Build history of the part. All positions in model axes, mm. A direction names the side the tool comes from. Give positions to 0.01 mm unless a question says otherwise; leave off trailing zeros. Loops run counter-clockwise (first coordinate to the right, second up) from the corner with the lowest first, then second, coordinate; pieces in that order, holes last. Notation, with made-up numbers: M 12.25,-24 L 52.25,-24 A29 cw 52.25,0 Z; hole C -38,-32.75 d10. An arc over 180 degrees is marked long. Answer as a JSON object with one key per item and string values. Group by question number.
1. Slice it at B-B (z = -64). List the corners of the cut face in (x, y).
2. Drop flat-ended pins along their axis: pin 1 Ø5 at (x, y) = (-1, 17.5) entering from -Z; pin 2 Ø8 at (y, z) = (1, -7.5) entering from -X; pin 3 Ø10.5 at (y, z) = (-20.5, -50.5) entering from +X; pin 4 Ø1 at (y, z) = (-5.5, -8.5) entering from +X. Give the stop position or say it passes through.
3. 3-axis set-ups, long thin cutter, end or side, ignore diameter. For faces 4 (the face through (6, -19, -54)), 5 (the face through (-3.525, -20.938, -54.072)), 6 (the face through (14, 0, 10)), 7 (the face through (-7.542, -23.397, -77.292)): which of +Z, -Z, +X, -X, +Y, -Y reach the whole face in a straight line?
4. Slice it at A-A (x = 20). List the corners of the cut face in (y, z), then the cut area to 3 significant figures.
5. Drill centre lines: line 1 along Z through (x, y) = (-4, -9.5); line 2 along X through (y, z) = (6.5, -2.5); line 3 along Z through (x, y) = (-21, -20.5). Where is each one in solid material? Low to high. Write a range as [from, to].
6. Mould opens along Z. For faces 1 (the face through (12.432, -8.508, -14.781)), 2 (the face through (-0.21, -10.896, -15.698)), 3 (the face through (25, 0, 0)) say: released by +Z, released by -Z, zero draft, split by the parting line, or undercut.
from build123d import *

# Parameters (mm, degrees)
BOSS_EXTRUDE1_DEPTH      = 25
BOSS_EXTRUDE1_DEPTH_BACK = 10
SKETCH1_R                = 10
SKETCH2_R                = 12.5
BOSS_EXTRUDE2_DEPTH      = 25
BOSS_EXTRUDE3_DEPTH      = 15
BOSS_EXTRUDE3_DEPTH_BACK = 15
CUT_EXTRUDE1_DEPTH       = 15
BOSS_EXTRUDE4_DEPTH      = 3.175
CUT_EXTRUDE2_DEPTH       = 96.96083651
CUT_EXTRUDE2_DEPTH_BACK  = 96.96083651
SKETCH10_R               = 5
CUT_EXTRUDE3_DEPTH       = 10


with BuildPart() as part:
    # Sketch1 → Boss-Extrude1 (new, two sides: drawn at the far end of the back side and taken through both)
    with BuildSketch(Plane(origin=(0, 0, 0), x_dir=(0, 0, -1), z_dir=(1, 0, 0)).offset(-BOSS_EXTRUDE1_DEPTH_BACK)):
        Circle(SKETCH1_R)
    extrude(amount=BOSS_EXTRUDE1_DEPTH + BOSS_EXTRUDE1_DEPTH_BACK)

    # Sketch2 → Boss-Extrude2 (add, symmetric)
    with BuildSketch(Plane(origin=(-10, 0, 0), x_dir=(0.9848069802426886, -0.173652560203633, 1.5808464272800858e-08), z_dir=(0.17364817766692736, 0.9847821256419462, -0.007104604780387524))):
        with Locations(Location((0, 0, 0), (0, 0, 180.000000906))):
            Circle(SKETCH2_R)
    extrude(amount=BOSS_EXTRUDE2_DEPTH, both=True)

    # Sketch5 → Boss-Extrude3 (add, two sides: drawn at the far end of the back side and taken through both)
    with BuildSketch(Plane(origin=(0, 0, 0), x_dir=(0, 0, -1), z_dir=(1, 0, 0)).offset(-BOSS_EXTRUDE3_DEPTH_BACK)):
        Polygon((0.79375, 1.374815329), (-0.79375, -1.374815329), (23.864525326, -15.611277226), (25.452025326, -12.861646569), align=None)
    extrude(amount=BOSS_EXTRUDE3_DEPTH + BOSS_EXTRUDE3_DEPTH_BACK)

    # Sketch6 → Cut-Extrude1 (cut)
    with BuildSketch(Plane(origin=(0, 1.374815329, -0.79375), x_dir=(1, 0, 0), z_dir=(0, 0.8660254037844419, -0.49999999999999434))):
        Polygon((15, 28.472923795), (15, 10), (8.276405599, 28.472923795), align=None)
    extrude(amount=-CUT_EXTRUDE1_DEPTH, mode=Mode.SUBTRACT)

    # Sketch8 → Boss-Extrude4 (add)
    with BuildSketch(Plane(origin=(0, -11.059465432, 1.950082148), x_dir=(1, 0, 0), z_dir=(0, 0.9848077530122095, -0.17364817766692275))):
        with BuildLine():
            Line((-15, 26.212839405), (8.276405599, 26.212839405))
            ThreePointArc((8.276405599, 26.212839405), (6.573986329, 32.197305321), (6, 38.392674831))
            Line((6, 38.392674831), (6, 76.212839405))
            ThreePointArc((6, 76.212839405), (-4.5, 65.712839405), (-15, 76.212839405))
            Line((-15, 76.212839405), (-15, 26.212839405))
        make_face()
        with BuildLine():
            ThreePointArc((6, 76.212839405), (-4.5, 86.712839405), (-15, 76.212839405))
            Line((-15, 76.212839405), (6, 76.212839405))
        make_face()
        with BuildLine():
            Line((6, 76.212839405), (-15, 76.212839405))
            ThreePointArc((-15, 76.212839405), (-4.5, 65.712839405), (6, 76.212839405))
        make_face()
    extrude(amount=BOSS_EXTRUDE4_DEPTH)

    # Sketch9 → Cut-Extrude2 (cut, two sides: drawn at the far end of the back side and taken through both)
    with BuildSketch(Plane(origin=(0, -7.932700816, 1.398749184), x_dir=(1, 0, 0), z_dir=(0, 0.9848077530122094, -0.173648177666923)).offset(-CUT_EXTRUDE2_DEPTH_BACK)):
        with BuildLine():
            Line((10.969458516, 56.012713561), (13.826274408, 16.792062616))
            ThreePointArc((13.826274408, 16.792062616), (6.0891037, 35.942860434), (10.969458516, 56.012713561))
        make_face()
    extrude(amount=CUT_EXTRUDE2_DEPTH + CUT_EXTRUDE2_DEPTH_BACK, mode=Mode.SUBTRACT)

    # Sketch10 → Cut-Extrude3 (cut)
    with BuildSketch(Plane(origin=(0, -7.932700816, 1.398749184), x_dir=(1, 0, 0), z_dir=(0, 0.9848077530122094, -0.17364817766692284))):
        with Locations(Location((-4.5, 76.212839405, 0), (0, 0, 270))):
            Circle(SKETCH10_R)
    extrude(amount=-CUT_EXTRUDE3_DEPTH, mode=Mode.SUBTRACT)


solid = part.part
Established:
{
 "1": {"outline": "M -15,-22.69 L 6,-22.69 L 6,-19.46 L -15,-19.46 Z"},
 "2": {"pin 1": "stops at z = -12.18", "pin 2": "stops at x = -22.18", "pin 3": "stops at x = 6", "pin 4": "stops at x = 25"},
 "3": {"face 4": "-Z, +X, +Y, -Y", "face 5": "+X, -X, -Y", "face 6": "+X", "face 7": "none"},
 "4": {"outline": "C 0,0 d20", "area": "314 mm^2"},
 "5": {"line 1": "z = [-19.63, -13.28], [-9.9, 10.02]", "line 2": "x = [-21.3, 25]", "line 3": "z = [-10.01, 10.32]"},
 "6": {"face 1": "released by -Z", "face 2": "undercut", "face 3": "zero draft"}
}
